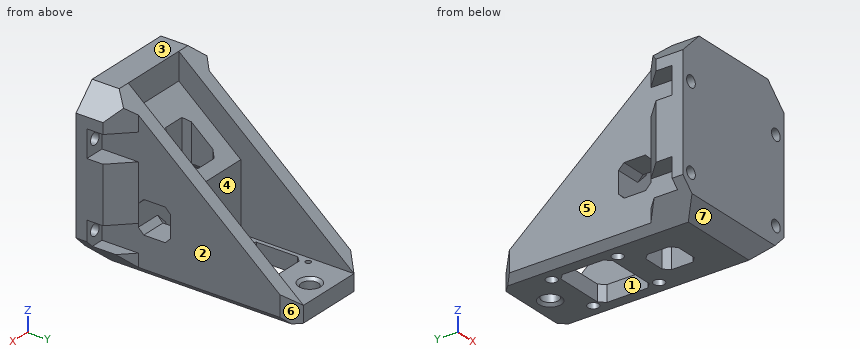
```python
from build123d import *

# Parameters (mm, degrees)
SKETCH1_W           = 50
SKETCH1_H           = 60
BOSS_EXTRUDE1_DEPTH = 10
SKETCH2_R           = 2.15
CUT_EXTRUDE1_DEPTH  = 4
SKETCH5_W           = 25
SKETCH5_H           = 6
BOSS_EXTRUDE3_DEPTH = 65
CUT_EXTRUDE3_REACH  = 101.247
SKETCH6_W           = 22
SKETCH6_H           = 19.25
SKETCH7_R           = 1
CUT_EXTRUDE4_DEPTH  = 2.5
CUT_EXTRUDE5_REACH  = 99.171
SKETCH8_R           = 2
BOSS_EXTRUDE4_DEPTH = 5
CHAMFER1_SIZE       = 7.5
CHAMFER2_SIZE       = 10
CHAMFER4_SIZE       = 5.5
CHAMFER5_SIZE       = 5
CHAMFER7_SIZE       = 2
CUT_EXTRUDE6_REACH  = 101.247
SKETCH10_R          = 3.1
CHAMFER8_SIZE       = 1
BOSS_EXTRUDE5_REACH = 91.058
CHAMFER9_SIZE       = 8
CUT_EXTRUDE7_REACH  = 101.247
SKETCH12_W          = 12
SKETCH12_H          = 12
CUT_EXTRUDE9_REACH  = 88.522
SKETCH14_W          = 12
SKETCH14_H          = 12
CHAMFER11_SIZE      = 2
CUT_EXTRUDE11_REACH = 93.276
SKETCH16_W          = 10
SKETCH16_H          = 13.5
SKETCH17_W          = 10
SKETCH17_H          = 13.5
CUT_EXTRUDE12_DEPTH = 7.5


# Some blends are built 0.0001 mm under size
with BuildPart() as part:
    # Sketch1 → Boss-Extrude1 (new body)
    with BuildSketch(Plane(origin=(0, 0, 0), x_dir=(1, 0, 0), z_dir=(0, 1, 0))):
        Rectangle(SKETCH1_W, SKETCH1_H)
    extrude(amount=BOSS_EXTRUDE1_DEPTH)

    # Sketch2 → Cut-Extrude1 (cut)
    with BuildSketch(Plane(origin=(0, 0, 0), x_dir=(1, 0, 0), z_dir=(0, 1, 0))):
        with Locations(Location((-21, 17.7, 0), (0, 0, 270))):
            Circle(SKETCH2_R)
        with Locations(Location((-21, -13, 0), (0, 0, 270))):
            Circle(SKETCH2_R)
        with Locations(Location((21, 17.7, 0), (0, 0, 270))):
            Circle(SKETCH2_R)
        with Locations(Location((21, -13, 0), (0, 0, 270))):
            Circle(SKETCH2_R)
    extrude(amount=CUT_EXTRUDE1_DEPTH, mode=Mode.SUBTRACT)

    # Sketch5 → Boss-Extrude3 (add)
    with BuildSketch(Plane(origin=(0, 10, 0), x_dir=(1, 0, 0), z_dir=(0, 1, 0))):
        with Locations((0, 27)):
            Rectangle(SKETCH5_W, SKETCH5_H)
    extrude(amount=BOSS_EXTRUDE3_DEPTH)

    # Sketch6 → Cut-Extrude3 (cut, up to next)
    with BuildSketch(Plane(origin=(0, 0, -30), x_dir=(-1, 0, 0), z_dir=(0, 0, -1)), mode=Mode.PRIVATE) as cut_extrude3_sk1:
        with Locations((0, 47.625)):
            Rectangle(SKETCH6_W, SKETCH6_H)
    cut_extrude3_tool1 = extrude(cut_extrude3_sk1.sketch, amount=-CUT_EXTRUDE3_REACH, mode=Mode.PRIVATE) & part.part
    add(cut_extrude3_tool1.solids().sort_by_distance((0, 47.625, -30))[0], mode=Mode.SUBTRACT)

    # Sketch7 → Cut-Extrude4 (cut)
    with BuildSketch(Plane.XY.offset(-24)):
        with Locations((10.25, 35.25)):
            Circle(SKETCH7_R)
        with Locations((-10.25, 35.25)):
            Circle(SKETCH7_R)
        with Locations((-10.25, 59.7)):
            Circle(SKETCH7_R)
        with Locations((10.25, 59.7)):
            Circle(SKETCH7_R)
    extrude(amount=-CUT_EXTRUDE4_DEPTH, mode=Mode.SUBTRACT)

    # Sketch8 → Cut-Extrude5 (cut, up to next)
    with BuildSketch(Plane.XY.offset(-26.5), mode=Mode.PRIVATE) as cut_extrude5_sk1:
        with Locations((-10.25, 59.7)):
            Circle(SKETCH8_R)
    cut_extrude5_tool1 = extrude(cut_extrude5_sk1.sketch, amount=-CUT_EXTRUDE5_REACH, mode=Mode.PRIVATE) & part.part
    # Sketch8 → Cut-Extrude5 (cut, up to next)
    with BuildSketch(Plane.XY.offset(-26.5), mode=Mode.PRIVATE) as cut_extrude5_sk2:
        with Locations((10.25, 59.7)):
            Circle(SKETCH8_R)
    cut_extrude5_tool2 = extrude(cut_extrude5_sk2.sketch, amount=-CUT_EXTRUDE5_REACH, mode=Mode.PRIVATE) & part.part
    # Sketch8 → Cut-Extrude5 (cut, up to next)
    with BuildSketch(Plane.XY.offset(-26.5), mode=Mode.PRIVATE) as cut_extrude5_sk3:
        with Locations((10.25, 35.25)):
            Circle(SKETCH8_R)
    cut_extrude5_tool3 = extrude(cut_extrude5_sk3.sketch, amount=-CUT_EXTRUDE5_REACH, mode=Mode.PRIVATE) & part.part
    # Sketch8 → Cut-Extrude5 (cut, up to next)
    with BuildSketch(Plane.XY.offset(-26.5), mode=Mode.PRIVATE) as cut_extrude5_sk4:
        with Locations((-10.25, 35.25)):
            Circle(SKETCH8_R)
    cut_extrude5_tool4 = extrude(cut_extrude5_sk4.sketch, amount=-CUT_EXTRUDE5_REACH, mode=Mode.PRIVATE) & part.part
    add(cut_extrude5_tool1.solids().sort_by_distance((-10.25, 59.7, -26.5))[0], mode=Mode.SUBTRACT)
    add(cut_extrude5_tool2.solids().sort_by_distance((10.25, 59.7, -26.5))[0], mode=Mode.SUBTRACT)
    add(cut_extrude5_tool3.solids().sort_by_distance((10.25, 35.25, -26.5))[0], mode=Mode.SUBTRACT)
    add(cut_extrude5_tool4.solids().sort_by_distance((-10.25, 35.25, -26.5))[0], mode=Mode.SUBTRACT)

    # Sketch9 → Boss-Extrude4 (add)
    with BuildSketch(Plane(origin=(12.5, 0, 0), x_dir=(0, 0, -1), z_dir=(1, 0, 0))):
        Polygon((30, 75), (24, 75), (-30, 10), (30, 10), align=None)
    boss_extrude4 = extrude(amount=BOSS_EXTRUDE4_DEPTH)

    # Mirror1: Boss-Extrude4 across plane
    add(boss_extrude4.mirror(Plane(origin=(0, 0, 0), x_dir=(0, 0, 1), z_dir=(1, 0, 0))))

    # Chamfer1
    chamfer1_edges = [part.edges().sort_by_distance(p)[0] for p in [
        (17.5, 10, 0),
        (-17.5, 10, 0),
    ]]
    chamfer(chamfer1_edges, length=CHAMFER1_SIZE - 0.0001)  # a hair under: the kernel refuses the full size

    # Chamfer2
    chamfer2_edges = [part.edges().sort_by_distance(p)[0] for p in [
        (-25, 5, -30),
        (25, 5, -30),
    ]]
    chamfer(chamfer2_edges, length=CHAMFER2_SIZE)

    # Chamfer4
    chamfer4_edges = [part.edges().sort_by_distance(p)[0] for p in [
        (0, 0, -30),
    ]]
    chamfer(chamfer4_edges, length=CHAMFER4_SIZE)

    # Chamfer5
    chamfer5_edges = [part.edges().sort_by_distance(p)[0] for p in [
        (17.5, 75, -25.75),
        (-17.5, 75, -25.75),
    ]]
    chamfer(chamfer5_edges, length=CHAMFER5_SIZE)

    # Chamfer7
    chamfer7_edges = [part.edges().sort_by_distance(p)[0] for p in [
        (-11, 57.25, -27),
        (-11, 38, -27),
        (11, 38, -27),
        (11, 57.25, -27),
    ]]
    chamfer(chamfer7_edges, length=CHAMFER7_SIZE)

    # Sketch10 → Cut-Extrude6 (cut, up to next)
    with BuildSketch(Plane(origin=(0, 0, -30), x_dir=(-1, 0, 0), z_dir=(0, 0, -1)), mode=Mode.PRIVATE) as cut_extrude6_sk1:
        with Locations((0, 68)):
            Circle(SKETCH10_R)
    cut_extrude6_tool1 = extrude(cut_extrude6_sk1.sketch, amount=-CUT_EXTRUDE6_REACH, mode=Mode.PRIVATE) & part.part
    add(cut_extrude6_tool1.solids().sort_by_distance((0, 68, -30))[0], mode=Mode.SUBTRACT)

    # Chamfer8
    chamfer8_edges = [part.edges().sort_by_distance(p)[0] for p in [
        (3.1, 68, -30),
        (3.1, 68, -24),
    ]]
    chamfer(chamfer8_edges, length=CHAMFER8_SIZE)

    # Sketch11 → Boss-Extrude5 (add, up to next)
    with BuildSketch(Plane(origin=(-12.5, 0, 0), x_dir=(0, 0, -1), z_dir=(1, 0, 0)), mode=Mode.PRIVATE) as boss_extrude5_sk1:
        Polygon((-20, 10), (24, 10), (24, 33), (-0.892307692, 33), align=None)
    boss_extrude5_tool1 = extrude(boss_extrude5_sk1.sketch, amount=BOSS_EXTRUDE5_REACH, mode=Mode.PRIVATE) - part.part
    add(boss_extrude5_tool1.solids().sort_by_distance((-12.5, 20.436802, -6.335287))[0])

    # Chamfer9
    # the kernel refuses this chamfer: 8 mm, written as the material it takes off along each edge
    with BuildSketch(Plane(origin=(25, -20.573463904, 30), x_dir=(0.027495876610586487, 0, -0.9996219169112968), z_dir=(0, 1, 0))) as chamfer9_piece_1:
        Polygon((CHAMFER9_SIZE * 0.999621916911, CHAMFER9_SIZE * 0.0274958766106), (-CHAMFER9_SIZE * 0.0274958766106, CHAMFER9_SIZE * 0.999621916911), (0, 0), align=None)
    extrude(amount=51.146927807, mode=Mode.SUBTRACT)
    with BuildSketch(Plane(origin=(-25, -20.573463904, 30), x_dir=(-0.027495876610586487, 0, -0.9996219169112968), z_dir=(0, 1, 0))) as chamfer9_piece_2:
        Polygon((CHAMFER9_SIZE * 0.999621916911, -CHAMFER9_SIZE * 0.0274958766106), (-CHAMFER9_SIZE * 0.0274958766106, -CHAMFER9_SIZE * 0.999621916911), (0, 0), align=None)
    extrude(amount=51.146927807, mode=Mode.SUBTRACT)

    # Cut-Extrude7: up to this plane
    cut_extrude7_end = Plane(origin=(25.002, 33, 0.892307692), z_dir=(0, -0.6390196945354668, -0.7691903730519506))
    # Sketch12 → Cut-Extrude7 (cut, up to the surface)
    with BuildSketch(Plane(origin=(0, 0, -30), x_dir=(-1, 0, 0), z_dir=(0, 0, -1)), mode=Mode.PRIVATE) as cut_extrude7_sk1:
        with Locations((0, 23.5)):
            Rectangle(SKETCH12_W, SKETCH12_H)
    cut_extrude7_tool1 = split(extrude(cut_extrude7_sk1.sketch, amount=-CUT_EXTRUDE7_REACH, mode=Mode.PRIVATE), bisect_by=cut_extrude7_end, keep=Keep.BOTH, mode=Mode.PRIVATE)
    add(cut_extrude7_tool1.solids().sort_by_distance((0, 23.5, -30))[0], mode=Mode.SUBTRACT)

    # Sketch14 → Cut-Extrude9 (cut, up to next)
    with BuildSketch(Plane(origin=(-6, 0, 0), x_dir=(0, 0, -1), z_dir=(1, 0, 0)), mode=Mode.PRIVATE) as cut_extrude9_sk1:
        with Locations((10, 23.5)):
            Rectangle(SKETCH14_W, SKETCH14_H)
    cut_extrude9_tool1 = extrude(cut_extrude9_sk1.sketch, amount=-CUT_EXTRUDE9_REACH, mode=Mode.PRIVATE) & part.part
    cut_extrude9 = cut_extrude9_tool1.solids().sort_by_distance((-6, 23.5, -10))[0]
    add(cut_extrude9, mode=Mode.SUBTRACT)

    # Mirror2: Cut-Extrude9 across plane
    add(cut_extrude9.mirror(Plane(origin=(0, 0, 0), x_dir=(0, 0, 1), z_dir=(1, 0, 0))), mode=Mode.SUBTRACT)

    # Chamfer11
    chamfer11_edges = [part.edges().sort_by_distance(p)[0] for p in [
        (-6, 17.5, 4.884615385),
        (6, 17.5, 4.884615385),
        (6, 29.5, -0.1),
        (-6, 29.5, -0.1),
        (-6, 17.5, -23),
        (-6, 29.5, -23),
        (-11.75, 17.5, -16),
        (-11.75, 29.5, -16),
        (-11.75, 17.5, -4),
        (-11.75, 29.5, -4),
        (-6, 23.5, -16),
        (-6, 23.5, -4),
        (6, 29.5, -23),
        (6, 17.5, -23),
        (11.75, 17.5, -4),
        (11.75, 17.5, -16),
        (6, 23.5, -16),
        (11.75, 29.5, -16),
        (11.75, 29.5, -4),
        (6, 23.5, -4),
    ]]
    chamfer(chamfer11_edges, length=CHAMFER11_SIZE)

    # Sketch16 → Cut-Extrude11 (cut, up to next)
    with BuildSketch(Plane(origin=(17.5, 0, 0), x_dir=(0, 0, -1), z_dir=(1, 0, 0)), mode=Mode.PRIVATE) as cut_extrude11_sk1:
        with Locations((-13, 10.75)):
            Rectangle(SKETCH16_W, SKETCH16_H)
    cut_extrude11_tool1 = extrude(cut_extrude11_sk1.sketch, amount=CUT_EXTRUDE11_REACH, mode=Mode.PRIVATE) & part.part
    cut_extrude11 = cut_extrude11_tool1.solids().sort_by_distance((17.5, 10.75, 13))[0]
    add(cut_extrude11, mode=Mode.SUBTRACT)

    # Sketch17 → Cut-Extrude12 (cut)
    with BuildSketch(Plane(origin=(17.5, 0, 0), x_dir=(0, 0, -1), z_dir=(1, 0, 0))):
        with Locations((17.7, 10.75)):
            Rectangle(SKETCH17_W, SKETCH17_H)
    cut_extrude12 = extrude(amount=CUT_EXTRUDE12_DEPTH, mode=Mode.SUBTRACT)

    # Mirror4: Cut-Extrude11, Cut-Extrude12 across plane
    add(cut_extrude11.mirror(Plane(origin=(0, 0, 0), x_dir=(0, 0, 1), z_dir=(1, 0, 0))), mode=Mode.SUBTRACT)
    add(cut_extrude12.mirror(Plane(origin=(0, 0, 0), x_dir=(0, 0, 1), z_dir=(1, 0, 0))), mode=Mode.SUBTRACT)


solid = part.part
```
Check sheet for the modelled part. Datum: model origin and axes. Units: mm. Face numbers are marked on the shaded views. A direction names the side the tool comes from. Give positions to 0.01 mm unless a question says otherwise; leave off trailing zeros. Write each loop counter-clockwise with the first axis right and the second up, starting at its lowest first coordinate (ties: lowest second). Pieces come first, ordered by that corner, then holes.
Item 1: Scan lines: L1, parallel to X at y = 1.15, z = 13; L2, parallel to X at y = 35, z = -28; L3, parallel to Y at x = 4, z = -14. Record each from-to range of solid material in increasing order.
Item 2: Gauge pin test, flat ends, axial feed: pin 1 (3 mm diameter, centred on x = -10.25, y = 59.7, fed in from -Z); pin 2 (4 mm diameter, centred on x = 21, y = 10, fed in from -Z); pin 3 (4 mm diameter, centred on x = -19.5, y = 7.5, fed in from +Z); pin 4 (2 mm diameter, centred on x = 0, z = 9, fed in from -Y). Record the tip position at first contact, or that the pin passes through.
Item 3: Cross-section at A-A (y = 45). Enter the section's corners in (x, z).
Item 4: Access from +Z, -Z, +X, -X, +Y, -Y to the whole of each face (thin tool, end or side, straight path). Record for the marked faces 1, 2, 3 and 4.
Item 5: Draft check along Z on the marked faces 5, 6 and 7. Enter one of: released by +Z, released by -Z, zero draft, split by the parting line, or undercut.
Item 6: Cross-section at C-C (y = 35.25). Enter the section's corners in (x, z), and give its area (3 significant figures).
Item 7: Cross-section at B-B (y = 25). Enter the section's corners in (x, z).
Report:
1. L1: x = -25 to -23.15, -18.85 to 18.85, 23.15 to 25
1. L2: x = -17 to -12.23, -8.27 to 8.27, 12.23 to 17
1. L3: y = 0 to 17.5, 29.5 to 33
2. pin 1: stops at z = -26.5
2. pin 2: stops at z = -26
2. pin 3: stops at z = 29.5
2. pin 4: stops at y = 0
3. outline: (-17.5, -27.5) - (-15, -30) - (-11, -30) - (-11, -24) - (-12.5, -24) - (-12.5, 0.92) - (-17.5, 0.92) - close; (11, -30) - (15, -30) - (17.5, -27.5) - (17.5, 0.92) - (12.5, 0.92) - (12.5, -24) - (11, -24) - close
4. face 1: +Z, -Z
4. face 2: +X, +Y
4. face 3: +Z, +X, -X, +Y, -Y
4. face 4: +Z, +Y
5. face 5: undercut
5. face 6: zero draft
5. face 7: released by -Z
6. outline: (-17.5, -27.5) - (-15, -30) - (-12.25, -30) - (-12.25, -26.5) - (-11.25, -26.5) - (-11.25, -24) - (-12.5, -24) - (-12.5, 9.02) - (-17.5, 9.02) - close; (-9.25, -26.5) - (-8.25, -26.5) - (-8.25, -30) - (8.25, -30) - (8.25, -26.5) - (9.25, -26.5) - (9.25, -24) - (-9.25, -24) - close; (11.25, -26.5) - (12.25, -26.5) - (12.25, -30) - (15, -30) - (17.5, -27.5) - (17.5, 9.02) - (12.5, 9.02) - (12.5, -24) - (11.25, -24) - close
6. area: 496 mm2
7. outline: (-17.5, -27.5) - (-15, -30) - (-6, -30) - (-6, -18) - (-8, -16) - (-17.5, -16) - close; (-17.5, -4) - (-8, -4) - (-6, -2) - (-6, 7.54) - (-12.5, 7.54) - (-12.5, 17.54) - (-17.5, 17.54) - close; (6, -30) - (15, -30) - (17.5, -27.5) - (17.5, -16) - (8, -16) - (6, -18) - close; (6, -2) - (8, -4) - (17.5, -4) - (17.5, 17.54) - (12.5, 17.54) - (12.5, 7.54) - (6, 7.54) - close
